Geometry check sheet. Reference: drawing and pictorial views, mm from the part's lowest x, y, z. A direction names the side the tool comes from. Round coordinates to 2 decimals unless told otherwise and drop trailing zeros. Order: outer loops, then holes, each group sorted by start corner. A loop starts at its lowest first (then second) coordinate and runs counter-clockwise, first axis right, second up.
(1) Sectioned sample at B-B (x = 39). Record the boundary of the cut face in (y, z).
(2) Material ranges on line 1 along Y through (x, z) = (39, 2); line 2 along X through (y, z) = (3, 33); line 3 along X through (y, z) = (3.25, 6.5), recorded low to high.
(3) Set-up check for the marked faces 1, 2, 3, 4 and 5: record each of +Z, -Z, +X, -X, +Y, -Y from which the full face is reachable in a straight line by a thin tool's end or side.
(4) Sectioned sample at A-A (z = 33). Record the boundary of the cut face in (x, y).
(5) Sectioned sample at D-D (y = 7). Record the boundary of the cut face in (x, z).
(6) Release check for a two-part mould opening along Z. For the marked faces 6, 7 and 8 record: +Z half, -Z half, draft (parallel to the pull), parting line (faces both ways), or undercut.
(7) Go/stop test with flat-tipped pins: pin 1 (2 mm diameter, centred on x = 11.5, y = 6.5, fed in from -Z); pin 2 (7 mm diameter, centred on x = 76.5, y = 4.5, fed in from -Z); pin 3 (2 mm diameter, centred on x = 4.5, y = 6, fed in from +Z). Record where each tip stops, or that it passes through.
(8) Sectioned sample at C-C (y = 12). Record the boundary of the cut face in (x, z), plus the area to 4 significant figures.
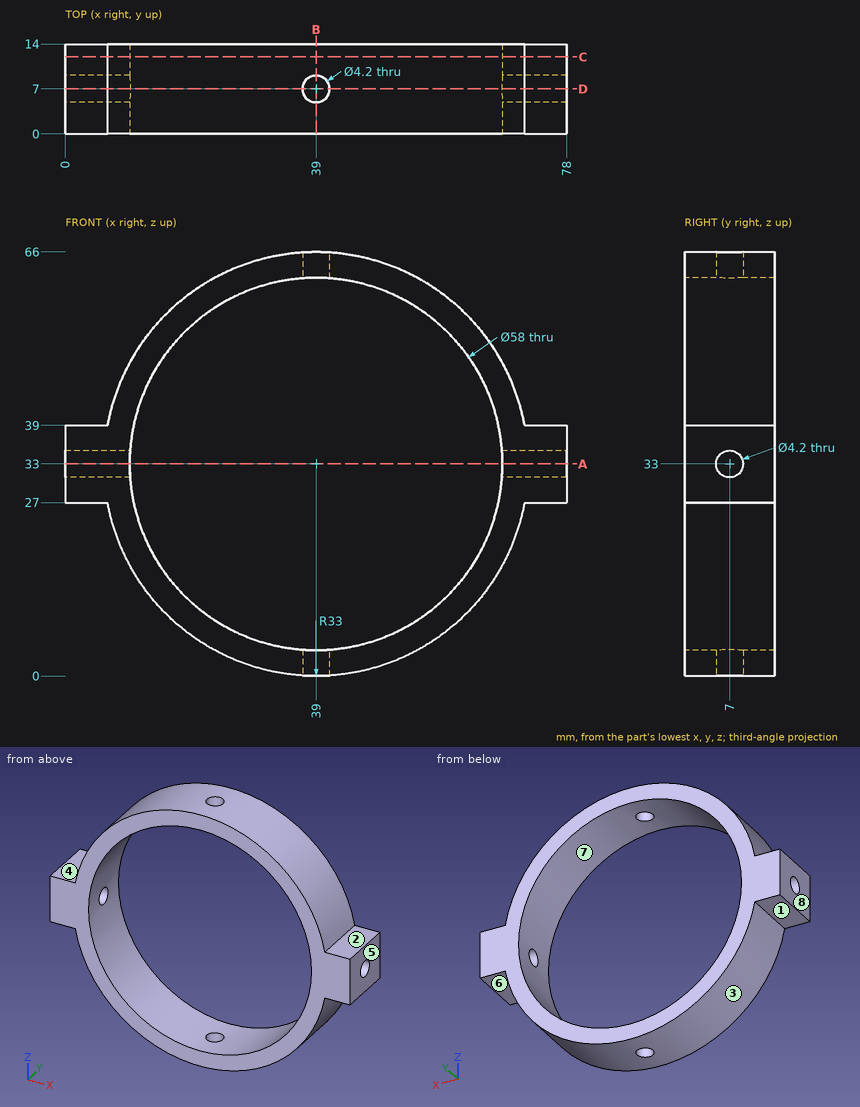
Answer below:
1. outline: (0, 0) - (4.9, 0) - (4.9, 4) - (0, 4) - close; (0, 62) - (4.9, 62) - (4.9, 66) - (0, 66) - close; (9.1, 0) - (14, 0) - (14, 4) - (9.1, 4) - close; (9.1, 62) - (14, 62) - (14, 66) - (9.1, 66) - close
2. line 1: y = 0 to 4.9, 9.1 to 14
2. line 2: x = 0 to 10, 68 to 78
2. line 3: x = 19.33 to 27.22, 50.78 to 58.67
3. face 1: -Z, -X, +Y, -Y
3. face 2: +Z, +X, +Y, -Y
3. face 3: -Z, +Y, -Y
3. face 4: +Z, -X, +Y, -Y
3. face 5: +Z, -Z, +X, +Y, -Y
4. outline: (0, 0) - (10, 0) - (10, 4.9) - (0, 4.9) - close; (0, 9.1) - (10, 9.1) - (10, 14) - (0, 14) - close; (68, 0) - (78, 0) - (78, 4.9) - (68, 4.9) - close; (68, 9.1) - (78, 9.1) - (78, 14) - (68, 14) - close
5. outline: (0, 27) - (6.55, 27) arc R33 ccw to (36.9, 0.07) - (36.9, 4.08) arc R29 cw to (10.08, 30.9) - (0, 30.9) - close; (0, 35.1) - (10.08, 35.1) arc R29 cw to (36.9, 61.92) - (36.9, 65.93) arc R33 ccw to (6.55, 39) - (0, 39) - close; (41.1, 0.07) arc R33 ccw to (71.45, 27) - (78, 27) - (78, 30.9) - (67.92, 30.9) arc R29 cw to (41.1, 4.08) - close; (41.1, 61.92) arc R29 cw to (67.92, 35.1) - (78, 35.1) - (78, 39) - (71.45, 39) arc R33 ccw to (41.1, 65.93) - close
6. face 6: -Z half
6. face 7: undercut
6. face 8: draft
7. pin 1: stops at z = 13.33
7. pin 2: stops at z = 27
7. pin 3: stops at z = 39
8. outline: (0, 27) - (6.55, 27) arc R33 ccw to (71.45, 27) - (78, 27) - (78, 39) - (71.45, 39) arc R33 ccw to (6.55, 39) - (0, 39) - close; hole circle Ø58 at (39, 33)
8. area: 927.5 mm2
